The model under review builds one solid part; all positions refer to its coordinate system, in mm. Coordinates: 2 decimals unless noted, no trailing zeros. Loops run counter-clockwise (first coordinate to the right, second up) from the corner with the lowest first, then second, coordinate; pieces in that order, holes last. Notation, with made-up numbers: M 59.25,37.25 L 69.25,37.25 A17 ccw 69.25,59.25 Z; hole C 87.25,23 d9. An arc over 180 degrees is marked long. Use CSV: the item, a comma, the result in double quotes. Start each with the question number.
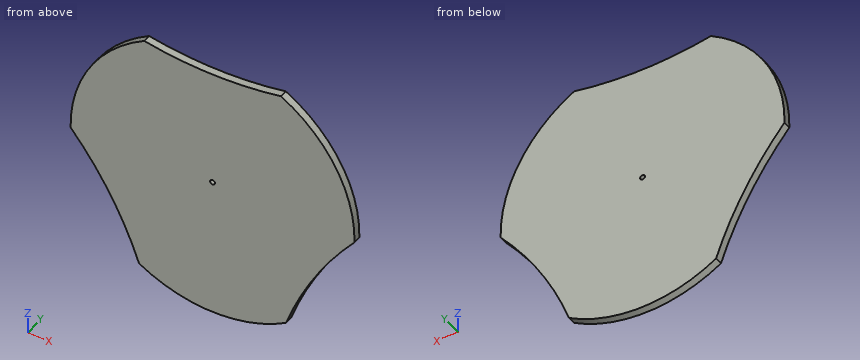
from build123d import *

# Parameters (mm, degrees)
SKETCH1_R           = 37
BOSS_EXTRUDE1_DEPTH = 1.6
SKETCH5_R           = 75.500139874
CUT_EXTRUDE2_DEPTH  = 2.6
SKETCH7_R           = 0.5
CUT_EXTRUDE3_DEPTH  = 2.6
SKETCH3_R           = 1.75
CUT_EXTRUDE4_DEPTH  = 2.6
SKETCH8_R           = 1.65
CUT_EXTRUDE5_DEPTH  = 2.6
CIRPATTERN2_COUNT   = 3
SKETCH10_OUTSIDE_W  = 94.454
SKETCH10_OUTSIDE_H  = 86.922
SKETCH10_OUTSIDE_R  = 29.5
CUT_EXTRUDE7_DEPTH  = 10


with BuildPart() as part:
    # Sketch1 → Boss-Extrude1 (new body)
    with BuildSketch(Plane(origin=(0, 0, 0), x_dir=(1, 0, 0), z_dir=(0, 1, 0))):
        Circle(SKETCH1_R)
    extrude(amount=BOSS_EXTRUDE1_DEPTH)

    # Sketch5 → Cut-Extrude2 (cut, through all)
    with BuildSketch(Plane(origin=(0, 1.6, 0), x_dir=(1, 0, 0), z_dir=(0, 1, 0))):
        with Locations((86.602540378, 50)):
            Circle(SKETCH5_R)
    cut_extrude2 = extrude(amount=-CUT_EXTRUDE2_DEPTH, mode=Mode.SUBTRACT)

    # Sketch7 → Cut-Extrude3 (cut, through all)
    with BuildSketch(Plane(origin=(0, 1.6, 0), x_dir=(1, 0, 0), z_dir=(0, 1, 0))):
        Circle(SKETCH7_R)
    extrude(amount=-CUT_EXTRUDE3_DEPTH, mode=Mode.SUBTRACT)

    # Sketch3 → Cut-Extrude4 (cut, through all)
    with BuildSketch(Plane(origin=(0, 1.6, 0), x_dir=(1, 0, 0), z_dir=(0, 1, 0))):
        with Locations((2.788983768, 31.878230339)):
            Circle(SKETCH3_R)
        with Locations((26.212865417, -18.354445963)):
            Circle(SKETCH3_R)
        with Locations((-29.001849185, -13.523784376)):
            Circle(SKETCH3_R)
    extrude(amount=-CUT_EXTRUDE4_DEPTH, mode=Mode.SUBTRACT)

    # Sketch8 → Cut-Extrude5 (cut, through all)
    with BuildSketch(Plane(origin=(0, 1.6, 0), x_dir=(1, 0, 0), z_dir=(0, 1, 0))):
        with Locations((-5.904038041, 33.483463602)):
            Circle(SKETCH8_R)
    cut_extrude5 = extrude(amount=-CUT_EXTRUDE5_DEPTH, mode=Mode.SUBTRACT)

    # CirPattern2: Cut-Extrude2, Cut-Extrude5 ×3 about axis
    cirpattern2_axis = Axis((0, 0, 0), (0, 1, 0))
    for i in range(1, CIRPATTERN2_COUNT):
        add(cut_extrude2.rotate(cirpattern2_axis, i * 360 / CIRPATTERN2_COUNT), mode=Mode.SUBTRACT)
        add(cut_extrude5.rotate(cirpattern2_axis, i * 360 / CIRPATTERN2_COUNT), mode=Mode.SUBTRACT)

    # Sketch10 outside → Cut-Extrude7 (cut)
    with BuildSketch(Plane(origin=(0, 1.6, 0), x_dir=(1, 0, 0), z_dir=(0, 1, 0))):
        with Locations((0, 4.328)):
            Rectangle(SKETCH10_OUTSIDE_W, SKETCH10_OUTSIDE_H)
        Circle(SKETCH10_OUTSIDE_R, mode=Mode.SUBTRACT)
    extrude(amount=-CUT_EXTRUDE7_DEPTH, mode=Mode.SUBTRACT)


solid = part.part
1. To check wall thickness, follow line 1 along Z through (x, y) = (0, 0.8); line 2 along X through (y, z) = (0.7, 0); line 3 along X through (y, z) = (0.2, 13.5). State the ranges of each line that lie inside material, in increasing order.
2. Add section B-B (z = -2.5). Write out the cut boundary in (x, y), plus the area to 3 significant figures.
3. Add section A-A (y = 0.6). Write out the cut boundary in (x, z), plus the area to 3 significant figures.
4. Add section C-C (x = 19.5). Write out the cut boundary in (y, z), plus the area to 3 significant figures.
Solved:
1,line 1,"z = -29.5 to -0.5, 0.5 to 24.5"
1,line 2,"x = -29.5 to -0.5, 0.5 to 29.5"
1,line 3,"x = -26.23 to 26.23"
2,outline,"M -27.92,0 L 27.92,0 L 27.92,1.6 L -27.92,1.6 Z"
2,area,"89.3 mm^2"
3,outline,"M -29.49,-0.62 A75.5 cw -15.28,-25.23 A29.5 ccw 15.28,-25.23 A75.5 cw 29.49,-0.62 A29.5 ccw 14.21,25.85 A75.5 cw -14.21,25.85 A29.5 ccw Z; hole C 0,0 d1"
3,area,"2,450 mm^2"
4,outline,"M 0,-15.39 L 1.6,-15.39 L 1.6,22.14 L 0,22.14 Z"
4,area,"60.0 mm^2"
